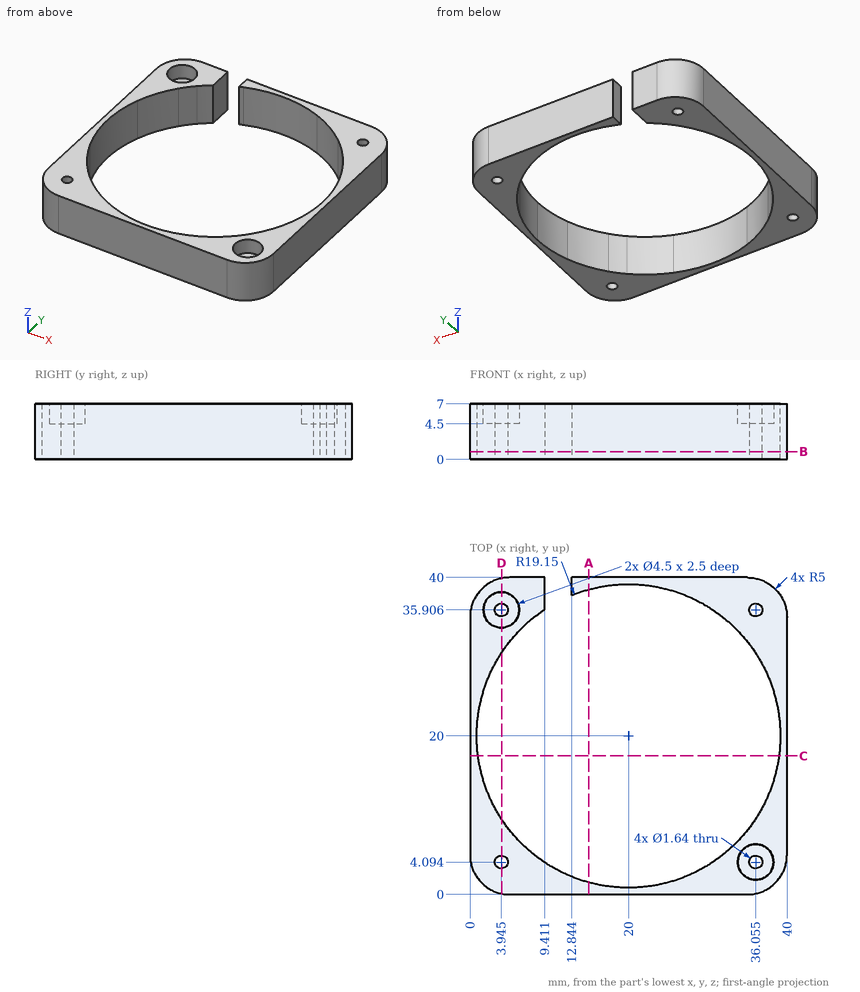
Check sheet for the drawn part. Datum: minimum x, y, z corner. Units: mm. Coordinates: 2 decimals unless noted, no trailing zeros. Write each loop counter-clockwise with the first axis right and the second up, starting at its lowest first coordinate (ties: lowest second). Pieces come first, ordered by that corner, then holes. Notation, with made-up numbers: (20.5, -0.75) - (38.5, -0.75) arc R14 cw to (38.5, 14.25) - close; hole circle Ø4 at (42.25, -34). An arc over 180 degrees is marked (long way). Answer as a JSON object with one key per item and string values.
(1) Cross-section at A-A on x = 15. Record the cut outline in (y, z) (1 decimal), plus the area to 3 significant figures.
Report:
{"outline": "(0, 0) - (1.5, 0) - (1.5, 7) - (0, 7) - close; (38.5, 0) - (40, 0) - (40, 7) - (38.5, 7) - close", "area": "21.2 mm^2"}
(2) Gauge pin test, flat ends, axial feed: pin 1 Ø1.3 at (x, y) = (4, 37) entering from +Z; pin 2 Ø2.5 at (x, y) = (3.94, 4.09) entering from -Z; pin 3 Ø1.1 at (y, z) = (39, 2.5) entering from -X. Record the tip position at first contact, or that the pin passes through.
Report:
{"pin 1": "z = 4.5", "pin 2": "z = 0", "pin 3": "x = 1.38"}
(3) Cross-section at B-B on z = 1. Give the number of separate pieces and of enclosed holes in the cut face.
Report:
{"separate pieces": "1", "enclosed holes": "4"}
(4) Cross-section at D-D on x = 4. Record the cut outline in (y, z) (1 decimal).
Report:
{"outline": "(0.1, 0) - (3.3, 0) - (3.3, 7) - (0.1, 7) - close; (4.9, 0) - (9.5, 0) - (9.5, 7) - (4.9, 7) - close; (30.5, 0) - (35.1, 0) - (35.1, 4.5) - (33.7, 4.5) - (33.7, 7) - (30.5, 7) - close; (36.7, 0) - (39.9, 0) - (39.9, 7) - (38.2, 7) - (38.2, 4.5) - (36.7, 4.5) - close"}
(5) Cross-section at C-C on y = 17.5. Record the cut outline in (x, z).
Report:
{"outline": "(0, 0) - (1.01, 0) - (1.01, 7) - (0, 7) - close; (38.99, 0) - (40, 0) - (40, 7) - (38.99, 7) - close"}
(6) Thickness scan on line 1 along Y through (x, z) = (19.5, 1.5); line 2 along X through (y, z) = (20, 5); line 3 along X through (y, z) = (3.5, 1.5). Record the ranges inside material, lowest first.
Report:
{"line 1": "0 to 0.86, 39.14 to 40", "line 2": "0 to 0.85, 39.15 to 40", "line 3": "0.23 to 3.38, 4.51 to 10.28, 29.72 to 35.49, 36.62 to 39.77"}
